```python
from build123d import *

# Parameters (mm, degrees)
ESBO_O1_R = 0.125


with BuildPart() as part:
    # Esboço1 → Revolução1 (revolve)
    with BuildSketch(Plane.XY, mode=Mode.PRIVATE) as revolu_o1_sk:
        with Locations((1, 7.868347502)):
            Circle(ESBO_O1_R)
        Polygon((1, 7.868347502), (1, 3.5), (0.25, 3.5), (0.25, 8), (0, 8), (2.344555434, 16.75), (16.5, 16.75), (16.5, 14.4), (13, 14.4), (13, 15.75), (3.111882422, 15.75), align=None)
    revolve(revolu_o1_sk.sketch.rotate(Axis((0, 0, 0), (1, 0, 0)), 90), axis=Axis((0, 0, 0), (1, 0, 0)))


solid = part.part
```
Input: part model. Units: mm. Frame: model coordinates. A direction names the side the tool comes from. Round coordinates to 2 decimals unless told otherwise and drop trailing zeros. Loops run counter-clockwise (first coordinate to the right, second up) from the corner with the lowest first, then second, coordinate; pieces in that order, holes last. Notation, with made-up numbers: (11, 82.25) -> (63, 82.25) arc R6 ccw to (63, 90.25) -> close; hole circle Ø7 at (33.25, -8.5). An arc over 180 degrees is marked (long way). Use one line per item in the form item = value. Start each with the question number.
Item 1: Contact query for flat-ended pins moving along their axis: pin 1 Ø1 at (x, z) = (11, -6.5) entering from +Y; pin 2 Ø3 at (x, z) = (4.5, 4) entering from -Y; pin 3 Ø4.5 at (y, z) = (1.5, 3) entering from +X; pin 4 Ø5.5 at (y, z) = (0, 0) entering from +X. Output: stop coordinate, or through.
Item 2: Set-up query: faces 1 (the face through (0.62, 3.105, 1.615)), 2 (the face through (1.133, 5.091, -6.639)), 3 (the face through (14.726, -4.325, 13.735)). Return all of +Z, -Z, +X, -X, +Y, -Y with unobstructed straight access to the full face (end or side cutting, diameter ignored); none if empty.
Item 3: Mould query, pull axis Z, two halves, no side actions, for faces 4 (the face through (7.987, -15.616, -2.05)), 5 (the face through (0.147, -2.567, 8.153)), 6 (the face through (16.5, -14, 5)), 7 (the face through (0.25, 1.7, -3.4)). Classes: pulls with the +Z half, pulls with the -Z half, needs draft (parallel to the pull), parting line crosses it, or undercut.
Item 4: Material intervals for L1, parallel to Z at x = 5.5, y = -8; L2, parallel to Y at x = 7.5, z = -2; L3, parallel to Y at x = 6, z = 8.5, sorted ascending. Write a range as from..to.
Item 5: Section query A-A on z = 0. Return the cut outline in (x, y) (3 decimals), then the cut area to 3 significant figures.
Ans:
q1.pin_1 = 15.64
q1.pin_2 = -16.56
q1.pin_3 = 1
q1.pin_4 = through
q2.face_1 = +X, -X
q2.face_2 = none
q2.face_3 = +X
q3.face_4 = undercut
q3.face_5 = parting line crosses it
q3.face_6 = needs draft
q3.face_7 = undercut
q4.L1 = -14.72..-13.57, 13.57..14.72
q4.L2 = -16.63..-15.62, 15.62..16.63
q4.L3 = -14.43..-13.26, 13.26..14.43
q5.outline = (0, -8) -> (2.345, -16.75) -> (16.5, -16.75) -> (16.5, -14.4) -> (13, -14.4) -> (13, -15.75) -> (3.112, -15.75) -> (1.032, -7.989) arc R0.125 ccw to (1, -7.743) -> (1, -3.5) -> (0.25, -3.5) -> (0.25, -8) -> close; (0, 8) -> (0.25, 8) -> (0.25, 3.5) -> (1, 3.5) -> (1, 7.743) arc R0.125 ccw to (1.032, 7.989) -> (3.112, 15.75) -> (13, 15.75) -> (13, 14.4) -> (16.5, 14.4) -> (16.5, 16.75) -> (2.345, 16.75) -> close
q5.area = 60.9 mm^2
